from build123d import *

# Parameters (mm, degrees)
ESQUISSE1_W             = 120
ESQUISSE1_H             = 100
BOSS_EXTRU_1_DEPTH      = 3
ESQUISSE2_W             = 2
ESQUISSE2_H             = 2
BOSS_EXTRU_2_DEPTH      = 3
ESQUISSE4_R             = 4
BOSS_EXTRU_4_DEPTH      = 70
ESQUISSE5_R             = 2
ENL_V_MAT_EXTRU_1_DEPTH = 70
CONG_1_R                = 10
BOSS_EXTRU_6_DEPTH      = 15
CONG_2_R                = 2


with BuildPart() as part:
    # Esquisse1 → Boss.-Extru.1 (new body)
    with BuildSketch(Plane(origin=(0, 0, 0), x_dir=(1, 0, 0), z_dir=(0, 1, 0))):
        with Locations((-60, 50)):
            Rectangle(ESQUISSE1_W, ESQUISSE1_H)
    extrude(amount=BOSS_EXTRU_1_DEPTH)

    # Esquisse2 → Boss.-Extru.2 (add)
    with BuildSketch(Plane(origin=(0, 3, 0), x_dir=(1, 0, 0), z_dir=(0, 1, 0))):
        Polygon((-105, 78), (-105, 80), (-103, 80), (-103, 82), (-107, 82), (-107, 78), align=None)
        Polygon((-105, 20), (-105, 22), (-107, 22), (-107, 18), (-103, 18), (-103, 20), align=None)
        Polygon((-43, 22), (-45, 22), (-45, 20), (-47, 20), (-47, 18), (-43, 18), align=None)
        Polygon((-47, 82), (-47, 80), (-45, 80), (-45, 78), (-43, 78), (-43, 82), align=None)
        with Locations((-6.8, 32.854127418)):
            Rectangle(ESQUISSE2_W, ESQUISSE2_H)
        with Locations((-6.8, 34.854127418)):
            Rectangle(ESQUISSE2_W, ESQUISSE2_H)
        with Locations((-8.8, 34.854127418)):
            Rectangle(ESQUISSE2_W, ESQUISSE2_H)
        with Locations((-27, 34.854127418)):
            Rectangle(ESQUISSE2_W, ESQUISSE2_H)
        with Locations((-29, 34.854127418)):
            Rectangle(ESQUISSE2_W, ESQUISSE2_H)
        with Locations((-29, 32.854127418)):
            Rectangle(ESQUISSE2_W, ESQUISSE2_H)
        with Locations((-29, 19.454127418)):
            Rectangle(ESQUISSE2_W, ESQUISSE2_H)
        with Locations((-29, 17.454127418)):
            Rectangle(ESQUISSE2_W, ESQUISSE2_H)
        with Locations((-27, 17.454127418)):
            Rectangle(ESQUISSE2_W, ESQUISSE2_H)
        with Locations((-5.8, 19.454127418)):
            Rectangle(ESQUISSE2_W, ESQUISSE2_H)
        with Locations((-5.8, 17.454127418)):
            Rectangle(ESQUISSE2_W, ESQUISSE2_H)
        with Locations((-7.8, 17.454127418)):
            Rectangle(ESQUISSE2_W, ESQUISSE2_H)
    extrude(amount=BOSS_EXTRU_2_DEPTH)

    # Esquisse4 → Boss.-Extru.4 (add)
    with BuildSketch(Plane(origin=(0, 3, 0), x_dir=(1, 0, 0), z_dir=(0, 1, 0))):
        with Locations((-10, 90)):
            Circle(ESQUISSE4_R)
        with Locations((-110, 90)):
            Circle(ESQUISSE4_R)
        with Locations((-110, 10)):
            Circle(ESQUISSE4_R)
        with Locations((-10, 10)):
            Circle(ESQUISSE4_R)
    extrude(amount=BOSS_EXTRU_4_DEPTH)

    # Esquisse5 → Enlèv. mat.-Extru.1 (cut)
    with BuildSketch(Plane(origin=(0, 73, 0), x_dir=(1, 0, 0), z_dir=(0, 1, 0))):
        with Locations((-110, 90)):
            Circle(ESQUISSE5_R)
        with Locations((-110, 10)):
            Circle(ESQUISSE5_R)
        with Locations((-10, 90)):
            Circle(ESQUISSE5_R)
        with Locations((-10, 10)):
            Circle(ESQUISSE5_R)
    extrude(amount=-ENL_V_MAT_EXTRU_1_DEPTH, mode=Mode.SUBTRACT)

    # Congé1
    cong_1_edges = [part.edges().sort_by_distance(p)[0] for p in [
        (0, 1.5, 0),
        (-120, 1.5, 0),
        (-120, 1.5, -100),
        (0, 1.5, -100),
    ]]
    fillet(cong_1_edges, radius=CONG_1_R)

    # Esquisse3 → Boss.-Extru.6 (add)
    with BuildSketch(Plane(origin=(0, 3, 0), x_dir=(1, 0, 0), z_dir=(0, 1, 0))):
        Polygon((-30, 78), (-28, 78), (-28, 80), (-23, 80), (-23, 78), (-21, 78), (-21, 82), (-28.2, 82), (-29.2, 82), (-30, 82), align=None)
        Polygon((-23, 63), (-28, 63), (-28, 65), (-30, 65), (-30, 61), (-26, 61), (-21, 61), (-21, 65), (-23, 65), align=None)
    extrude(amount=BOSS_EXTRU_6_DEPTH)

    # Congé2
    cong_2_edges = [part.edges().sort_by_distance(p)[0] for p in [
        (-30, 4.5, -16.454127418),
        (-4.8, 4.5, -16.454127418),
        (-107, 4.5, -82),
        (-21, 10.5, -82),
        (-30, 10.5, -82),
        (-30, 10.5, -61),
        (-21, 10.5, -61),
        (-107, 4.5, -18),
        (-43, 4.5, -18),
        (-43, 4.5, -82),
        (-5.8, 4.5, -35.854127418),
        (-30, 4.5, -35.854127418),
    ]]
    fillet(cong_2_edges, radius=CONG_2_R)


solid = part.part
Design review of the part built by this model. Coordinates are the model's own, in mm. A direction names the side the tool comes from. Coordinates: 2 decimals unless noted, no trailing zeros. Loops run counter-clockwise (first coordinate to the right, second up) from the corner with the lowest first, then second, coordinate; pieces in that order, holes last. Notation, with made-up numbers: (59.25, 74) - (112.25, 74) arc R23 ccw to (112.25, 93) - close; hole circle Ø2 at (-4, 45.25). An arc over 180 degrees is marked (long way). Use CSV: the item, a comma, the result in double quotes. Start each with the question number.
1. For faces 5 (the flat face through (-45, 6, -80.5)), 6 (the flat face through (-12, 73, -9)), 7 (the flat face through (-10, 3, -10)), 8 (the flat face through (-105.5, 6, -20)), 9 (the flat face through (-61, 0, -51)), list the 3-axis set-ups (+Z, -Z, +X, -X, +Y, -Y) from which the entire face can be reached by the end or side of a thin tool; tool diameter is ignored.
2. Add section D-D on z = -73.5. Give the boundary of the cut face in (x, y), plus the area to 3 significant figures.
3. Clearance check with flat-ended pins moving along their axes: pin 1 (0.6 mm diameter, centred on x = -29, y = 8, fed in from +Z); pin 2 (1.6 mm diameter, centred on x = -27.5, y = 5, fed in from -Z); pin 3 (0.6 mm diameter, centred on y = 4, z = -32.5, fed in from -X). State where each tip first meets the part, or that it passes through.
4. Add section B-B on y = 24. Give the boundary of the cut face in (x, z), plus the area to 3 significant figures.
5. Add section C-C on x = -77.5. Give the boundary of the cut face in (y, z), plus the area to 3 significant figures.
6. To check wall thickness, follow probe 1 along X at (y, z) = (24, -10); probe 2 along Z at (x, y) = (-110, 53); probe 3 along Y at (x, z) = (-91, -61). State the ranges of each line that lie inside material, in increasing order.
7. Mouldability with a two-part tool opening along Z and no side actions: class faces 1 (the cylindrical face through (-110, 38, -92)), 2 (the cylindrical face through (-117.15, 1.52, -3.01)), 3 (the flat face through (-25, 10, -82)), 4 (the flat face through (-44.6, 6, -19.6)) as released by +Z, released by -Z, zero draft, split by the parting line, or undercut.
8. Add section A-A on y = 14.5. Count the separate pieces of the cut face and the enclosed holes in it, plus the area to 3 significant figures.
Resolved:
1,face 5,"+Z, -Z, -X, +Y"
1,face 6,"+Z, -Z, +X, -X, +Y"
1,face 7,"+Y"
1,face 8,"+X, -X, +Y"
1,face 9,"+Z, -Z, +X, -X, -Y"
2,outline,"(-120, 0) - (0, 0) - (0, 3) - (-120, 3) - close"
2,area,"360 mm2"
3,pin 1,"z = -61.13"
3,pin 2,"z = -82"
3,pin 3,"x = -30"
4,outline,"circle Ø8 at (-110, -90); circle Ø8 at (-110, -10); circle Ø8 at (-10, -90); circle Ø8 at (-10, -10); hole circle Ø4 at (-110, -90); hole circle Ø4 at (-110, -10); hole circle Ø4 at (-10, -90); hole circle Ø4 at (-10, -10)"
4,area,"151 mm2"
5,outline,"(0, -100) - (3, -100) - (3, 0) - (0, 0) - close"
5,area,"300 mm2"
6,probe 1,"-114 to -112, -108 to -106, -14 to -12, -8 to -6"
6,probe 2,"-94 to -92, -88 to -86, -14 to -12, -8 to -6"
6,probe 3,"0 to 3"
7,face 1,"undercut"
7,face 2,"released by +Z"
7,face 3,"released by -Z"
7,face 4,"zero draft"
8,separate pieces,"6"
8,enclosed holes,"4"
8,area,"199 mm2"
